Work out the finished part from the listing and answer in its coordinate system (mm). A direction names the side the tool comes from. Round coordinates to 2 decimals unless told otherwise and drop trailing zeros. Loops run counter-clockwise (first coordinate to the right, second up) from the corner with the lowest first, then second, coordinate; pieces in that order, holes last. Notation, with made-up numbers: M -24,53.25 L 3,53.25 A17 cw 3,73.25 Z; hole C 41,-24 d2. An arc over 180 degrees is marked long. One line per item, written item: value.
```python
from build123d import *
from build123d.topology import SkipClean

# Parameters (mm, degrees)
SKETCH2_R           = 8
BOSS_EXTRUDE1_DEPTH = 18
BOSS_EXTRUDE3_DEPTH = 9
FILLET1_R           = 0.4
SKETCH12_R          = 1.1
CUT_EXTRUDE2_DEPTH  = 30.274562429
SKETCH13_R          = 1.7
CUT_EXTRUDE3_DEPTH  = 31.055691415
SKETCH14_W          = 4.5
SKETCH14_H          = 5.58
BOSS_EXTRUDE5_DEPTH = 6
SKETCH15_R          = 1.7
CUT_EXTRUDE4_DEPTH  = 33.143110095
SKETCH18_RX         = 2.125
SKETCH18_RY         = 1.56360128
CUT_EXTRUDE5_DEPTH  = 27.532998323
BOSS_EXTRUDE6_START = 11
BOSS_EXTRUDE6_DEPTH = 11
CUT_EXTRUDE6_DEPTH  = 3.5


with BuildPart() as part:
    # Sketch2 → Boss-Extrude1 (new body)
    with BuildSketch(Plane(origin=(0, 0, 0), x_dir=(1, 0, 0), z_dir=(0, 1, 0))):
        with Locations(Location((0, 0, 0), (0, 0, 270))):
            Circle(SKETCH2_R)
    extrude(amount=BOSS_EXTRUDE1_DEPTH)

    # Sketch4 → Boss-Extrude3 (add)
    with BuildSketch(Plane(origin=(0, 18, 0), x_dir=(1, 0, 0), z_dir=(0, 1, 0))):
        with BuildLine():
            Line((2.504502892, -1.8), (2.504502892, 1.8))
            ThreePointArc((2.504502892, 1.8), (0, 3.30267653), (-2.504502892, 1.8))
            Line((-2.504502892, 1.8), (-2.504502892, -1.8))
            ThreePointArc((-2.504502892, -1.8), (0, -3.30267653), (2.504502892, -1.8))
        make_face()
    extrude(amount=BOSS_EXTRUDE3_DEPTH)

    # Fillet1
    fillet1_edges = [part.edges().sort_by_distance(p)[0] for p in [
        (0, 18, -3.30267653),
        (0, 18, 3.30267653),
    ]]
    fillet(fillet1_edges, radius=FILLET1_R)

    # Sketch12 → Cut-Extrude2 (cut, through all)
    with BuildSketch(Plane(origin=(0, 0, 0), x_dir=(1, 0, 0), z_dir=(0, 1, 0))):
        with Locations(Location((0, 5.887857779, 0), (0, 0, 270))):
            Circle(SKETCH12_R)
    extrude(amount=CUT_EXTRUDE2_DEPTH, mode=Mode.SUBTRACT)

    # Sketch13 → Cut-Extrude3 (cut, through all)
    with BuildSketch(Plane.ZY.offset(2.504502892)):
        with Locations((0, 24.5)):
            Circle(SKETCH13_R)
    extrude(amount=-CUT_EXTRUDE3_DEPTH, mode=Mode.SUBTRACT)

    # Sketch14 → Boss-Extrude5 (add)
    with BuildSketch(Plane.XZ):
        with Locations((-5.247726322, 0)):
            Rectangle(SKETCH14_W, SKETCH14_H)
        with Locations((5.247726322, 0)):
            Rectangle(SKETCH14_W, SKETCH14_H)
    extrude(amount=BOSS_EXTRUDE5_DEPTH)

    # Sketch15 → Cut-Extrude4 (cut, through all)
    with BuildSketch(Plane(origin=(7.497726322, 0, 0), x_dir=(0, 0, -1), z_dir=(1, 0, 0))):
        with Locations((0, -3)):
            Circle(SKETCH15_R)
    extrude(amount=-CUT_EXTRUDE4_DEPTH, mode=Mode.SUBTRACT)

    # Sketch18 → Cut-Extrude5 (cut, through all)
    with BuildSketch(Plane(origin=(0, 18, 0), x_dir=(1, 0, 0), z_dir=(0, 1, 0))):
        with Locations(Location((0, -5.788604863), (0, 0, 180))):
            Ellipse(SKETCH18_RX, SKETCH18_RY)
    extrude(amount=-CUT_EXTRUDE5_DEPTH, mode=Mode.SUBTRACT)

    # Sketch19 → Boss-Extrude6 (add)
    with SkipClean():  # the faces are left unmerged after this step: merging them gives an invalid solid
        with BuildSketch(Plane.XZ.offset(BOSS_EXTRUDE6_START)):
            with BuildLine():
                Line((-6.832550312, 4.1612806), (-4.998986356, 3.04457106))
                ThreePointArc((-4.998986356, 3.04457106), (-3.54196191, 3.971164487), (-2.080323071, 4.890461784))
                Line((-2.080323071, 4.890461784), (-3.131517904, 7.361629956))
                ThreePointArc((-3.131517904, 7.361629956), (-5.232707029, 6.051345069), (-6.832550312, 4.1612806))
            make_face()
            with BuildLine():
                Line((3.131517904, 7.361629956), (2.080323071, 4.890461784))
                ThreePointArc((2.080323071, 4.890461784), (3.54196191, 3.971164487), (4.998986356, 3.04457106))
                Line((4.998986356, 3.04457106), (6.832550312, 4.1612806))
                ThreePointArc((6.832550312, 4.1612806), (5.232707029, 6.051345069), (3.131517904, 7.361629956))
            make_face()
        extrude(amount=-BOSS_EXTRUDE6_DEPTH)

    # Sketch20 → Cut-Extrude6 (cut)
    with SkipClean():  # the faces are left unmerged after this step: merging them gives an invalid solid
        with BuildSketch(Plane.XZ):
            Polygon((2.911854561, -2.79), (2.911854561, 2.79), (2.911854561, 4.372678458), (-2.997726322, 4.372678458), (-2.997726322, 2.79), (-2.997726322, -2.79), (-2.997726322, -4.306263787), (2.911854561, -4.306263787), align=None)
        extrude(amount=-CUT_EXTRUDE6_DEPTH, mode=Mode.SUBTRACT)


solid = part.part
```
1) Find section C-C (z = -6.5). Give the vertices of the cut face in (x, y).
Check values:
outline: M -4.66,0 L -0.91,0 L -0.91,18 L -4.66,18 Z; M 0.91,0 L 4.66,0 L 4.66,18 L 0.91,18 Z
2) Find section B-B (y = -3). Give the vertices of the cut face in (x, z).
Check values:
outline: M -7.5,-2.79 L -3,-2.79 L -3,-1.7 L -7.5,-1.7 Z; M -7.5,1.7 L -3,1.7 L -3,2.79 L -7.5,2.79 Z; M -6.83,4.16 L -5,3.04 A345.37 cw -2.08,4.89 L -3.13,7.36 A8 ccw Z; M 2.08,4.89 A345.37 cw 5,3.04 L 6.83,4.16 A8 ccw 3.13,7.36 Z; M 3,-2.79 L 7.5,-2.79 L 7.5,-1.7 L 3,-1.7 Z; M 3,1.7 L 7.5,1.7 L 7.5,2.79 L 3,2.79 Z
3) Each of these flat-tipped pins is pushed along its axis until it touches: pin 1 (5 mm diameter, centred on x = -5, y = -4.5, fed in from -Z); pin 2 (5 mm diameter, centred on x = 5, z = 0.5, fed in from -Y); pin 3 (5 mm diameter, centred on x = -2.5, z = 6, fed in from +Y). Where does it stop, or does it pass through?
Check values:
pin 1: z = -2.79
pin 2: y = -6
pin 3: y = 18
4) Find section A-A (z = 0). Give the number of separate pieces and of enclosed holes in the cut face, then the cut area to 3 significant figures.
Check values:
separate pieces: 4
enclosed holes: 0
area: 319 mm2
5) For faces 1 (the face through (5, -6, 0)), 2 (the face through (0.043, 22.64, -3.302)), 3 (the face through (-7.498, -1.6, -1.3)), 4 (the face through (7.498, -1.6, -1.3)), 5 (the face through (-2.505, 21, 0)), determine the directions among +Z, -Z, +X, -X, +Y, -Y from which every point of the face is accessible in a straight line to the end or side of a thin tool.
Check values:
face 1: -Z, +X, -X, -Y
face 2: -Z, +Y
face 3: +Z, -Z, -X, -Y
face 4: +Z, -Z, +X, -Y
face 5: +Z, -Z, -X, +Y
6) Find the intervals of material crossed by probe 1 along Y at (x, z) = (4.1, 0); probe 2 along Y at (x, z) = (-2.5, 6.75); probe 3 along Y at (x, z) = (-2.5, 3.5), in increasing order. Write a range as from..to.
Check values:
probe 1: -6..-4.7, -1.3..18
probe 2: 0..18
probe 3: 3.5..18
7) The mould has two halves that part along Z. Classify faces 6 (the face through (-2.998, 0, 0)), 7 (the face through (0, 0, 7.8)), 8 (the face through (2.61, -5.58, 6.14)): +Z half, -Z half, draft (parallel to the pull), parting line (faces both ways), or undercut.
Check values:
face 6: undercut
face 7: draft
face 8: +Z half
